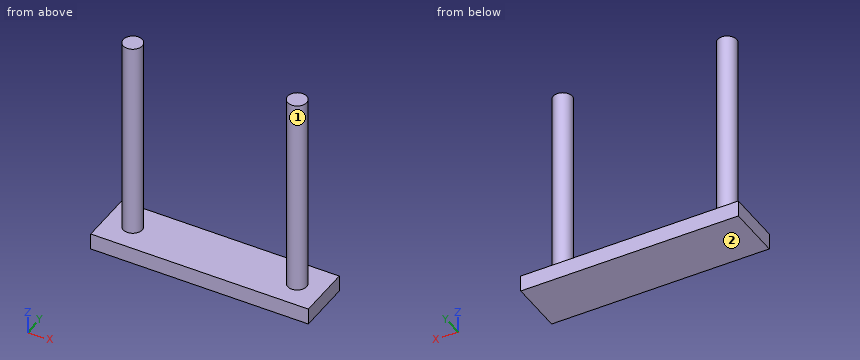
```python
from build123d import *

# Parameters (mm, degrees)
F0_R     = 1.75
F1_DEPTH = 3
F2_DEPTH = 40


with BuildPart() as f1:
    # F0 (on Top) → F1 (new body)
    with BuildSketch(Plane.XY):
        Polygon((3.954127, 14.839267), (-16.045873, 14.839267), (-16.045873, 4.839267), (3.954127, 4.839267), (23.954127, 4.839267), (23.954127, 14.839267), align=None)
        with Locations((-11.157998, 9.839267)):
            Circle(F0_R, mode=Mode.SUBTRACT)
        with Locations((19.066252, 9.839267)):
            Circle(F0_R, mode=Mode.SUBTRACT)
    extrude(amount=F1_DEPTH)

    # F0 (on Top) → F2 (join)
    with BuildSketch(Plane.XY):
        with Locations((19.066252, 9.839267)):
            Circle(F0_R)
        with Locations((-11.157998, 9.839267)):
            Circle(F0_R)
    extrude(amount=F2_DEPTH)


solid = f1.part
```
Could you check a few things on this model? Use its own coordinates, in mm. Face numbers are marked on the shaded views. Round coordinates to 2 decimals unless told otherwise and drop trailing zeros. Order: outer loops, then holes, each group sorted by start corner. A loop starts at its lowest first (then second) coordinate and runs counter-clockwise, first axis right, second up. Notation, with made-up numbers: M 89,45.5 L 109,45.5 A22 ccw 109,76.5 Z; hole C 7.5,-8 d1. An arc over 180 degrees is marked long. One line per question, with ' | ' between items. Start each with the question number.
(1) For P1, Ø8, axis at x = 10.5, z = 14, coming from the -Y side; P2, Ø3, axis at x = 8.5, y = 8.5, coming from the +Z side; P3, Ø1, axis at y = 11.5, z = 8.5, coming from the +X side, each with a flat end and sliding along its axis, tell me the tip position at first contact or that it passes through.
(2) Suppose I cut it at A-A on y = 9. List the corners of the cut face in (x, z) for me, then the cut area to 3 significant figures.
(3) Please list where these lines run through material, in increasing order: line 1 along Z through (x, y) = (-13.5, 6); line 2 along X through (y, z) = (9.5, 7); line 3 along X through (y, z) = (10.75, 8).
(4) Suppose I cut it at D-D on y = 13.5. List the corners of the cut face in (x, z) for me.
(5) Suppose I cut it at C-C on z = 5.5. List the corners of the cut face in (x, y) for me.
(6) Thinking about a two-plate mould opening in X: for the marked faces 1 and 2, which applies, +X half, -X half, draft (parallel to the pull), parting line (faces both ways), or undercut?
(7) Suppose I cut it at B-B on x = 13. List the corners of the cut face in (y, z) for me.
Geometry results:
1) P1: through | P2: z = 3 | P3: x = 20.38
2) outline: M -16.05,0 L 23.95,0 L 23.95,3 L 20.6,3 L 20.6,40 L 17.53,40 L 17.53,3 L -9.62,3 L -9.62,40 L -12.69,40 L -12.69,3 L -16.05,3 Z | area: 347 mm²
3) line 1: 0 to 3 | line 2: -12.87 to -9.44, 17.35 to 20.78 | line 3: -12.65 to -9.66, 17.57 to 20.56
4) outline: M -16.05,0 L 23.95,0 L 23.95,3 L -16.05,3 Z
5) outline: C -11.16,9.84 d3.5; C 19.07,9.84 d3.5
6) face 1: undercut | face 2: draft
7) outline: M 4.84,0 L 14.84,0 L 14.84,3 L 4.84,3 Z
